Check sheet for the modelled part. Datum: model origin and axes. Units: mm. A direction names the side the tool comes from. Round coordinates to 2 decimals unless told otherwise and drop trailing zeros. Loops run counter-clockwise (first coordinate to the right, second up) from the corner with the lowest first, then second, coordinate; pieces in that order, holes last. Notation, with made-up numbers: (62.25, 62.25) - (79.25, 62.25) arc R28 ccw to (79.25, 91.25) - close; hole circle Ø3 at (71, 63.5). An arc over 180 degrees is marked (long way). Return JSON: item names as keys, results as strings.
from build123d import *

# Parameters (mm, degrees)
F0_W     = 45.085
F0_H     = 62.992
F1_DEPTH = 25.654
F2_R     = 2.286
F3_DEPTH = 35.306
F5_DEPTH = 21.209
F6_W     = 10.668
F6_H     = 7.9248
F7_DEPTH = 11.43
F8_W     = 10.668
F8_H     = 7.9248
F9_DEPTH = 11.43


with BuildPart() as f1:
    # F0 (on Front) → F1 (new body)
    with BuildSketch(Plane.XZ):
        Rectangle(F0_W, F0_H)
    extrude(amount=F1_DEPTH)

    # F2 (on face) → F3 (cut)
    with BuildSketch(Plane.XZ.offset(25.654)):
        with Locations((0, 23.876)):
            Circle(F2_R)
        with BuildLine():
            Line((-2.2225, -22.7965), (-2.2225, -25.4635))
            ThreePointArc((-2.2225, -25.4635), (0, -27.686), (2.2225, -25.4635))
            Line((2.2225, -25.4635), (2.2225, -22.7965))
            ThreePointArc((2.2225, -22.7965), (0, -20.574), (-2.2225, -22.7965))
        make_face()
    extrude(amount=-F3_DEPTH, mode=Mode.SUBTRACT)

    # F4 (on face) → F5 (cut)
    with BuildSketch(Plane.XZ.offset(25.654)):
        with BuildLine():
            Line((-5.08, 34.951579), (-5.08, 23.876))
            ThreePointArc((-5.08, 23.876), (0, 18.796), (5.08, 23.876))
            Line((5.08, 23.876), (5.08, 34.951579))
            Line((5.08, 34.951579), (-5.08, 34.951579))
        make_face()
        with BuildLine():
            Line((5.08, -34.4517), (5.08, -24.13))
            ThreePointArc((5.08, -24.13), (0, -19.05), (-5.08, -24.13))
            Line((-5.08, -24.13), (-5.08, -34.4517))
            Line((-5.08, -34.4517), (5.08, -34.4517))
        make_face()
    extrude(amount=-F5_DEPTH, mode=Mode.SUBTRACT)

    # F6 (on face) → F7 (cut)
    with BuildSketch(Plane(origin=(0, 0, -31.496), x_dir=(1, 0, 0), z_dir=(0, 0, -1))):
        with Locations((-13.716, 19.1516)):
            Rectangle(F6_W, F6_H)
        with Locations((13.716, 19.1516)):
            Rectangle(F6_W, F6_H)
    extrude(amount=-F7_DEPTH, mode=Mode.SUBTRACT)

    # F8 (on face) → F9 (cut)
    with BuildSketch(Plane.XY.offset(31.496)):
        with Locations((13.716, -19.1516)):
            Rectangle(F8_W, F8_H)
        with Locations((-13.716, -19.1516)):
            Rectangle(F8_W, F8_H)
    extrude(amount=-F9_DEPTH, mode=Mode.SUBTRACT)


solid = f1.part
Q1. Sectioned sample at C-C (x = 15). Enter the section's corners in (y, z).
Answer key:
{"outline": "(-25.65, -31.5) - (-23.11, -31.5) - (-23.11, -20.07) - (-15.19, -20.07) - (-15.19, -31.5) - (0, -31.5) - (0, 31.5) - (-15.19, 31.5) - (-15.19, 20.07) - (-23.11, 20.07) - (-23.11, 31.5) - (-25.65, 31.5) - close"}
Q2. Sectioned sample at D-D (y = -20.25). Enter the section's corners in (x, z).
Answer key:
{"outline": "(-22.54, -31.5) - (-19.05, -31.5) - (-19.05, -20.07) - (-8.38, -20.07) - (-8.38, -31.5) - (-5.08, -31.5) - (-5.08, -24.13) arc R5.08 cw to (5.08, -24.13) - (5.08, -31.5) - (8.38, -31.5) - (8.38, -20.07) - (19.05, -20.07) - (19.05, -31.5) - (22.54, -31.5) - (22.54, 31.5) - (19.05, 31.5) - (19.05, 20.07) - (8.38, 20.07) - (8.38, 31.5) - (5.08, 31.5) - (5.08, 23.88) arc R5.08 cw to (-5.08, 23.88) - (-5.08, 31.5) - (-8.38, 31.5) - (-8.38, 20.07) - (-19.05, 20.07) - (-19.05, 31.5) - (-22.54, 31.5) - close"}
Q3. Scan lines: probe 1 along Z at (x, y) = (0, -2.35); probe 2 along X at (y, z) = (-23, -25.5); probe 3 along X at (y, z) = (-5.75, 28.5). Record each from-to range of solid material in increasing order. Write a range as [from, to].
Answer key:
{"probe 1": "z = [-31.5, -27.69], [-20.57, 21.59], [26.16, 31.5]", "probe 2": "x = [-22.54, -19.05], [-8.38, -5.08], [5.08, 8.38], [19.05, 22.54]", "probe 3": "x = [-22.54, -5.08], [5.08, 22.54]"}
Q4. Sectioned sample at A-A (x = 0). Enter the section's corners in (y, z) (3 decimals).
Answer key:
{"outline": "(-25.654, -19.05) - (-4.445, -19.05) - (-4.445, -20.574) - (0, -20.574) - (0, 21.59) - (-4.445, 21.59) - (-4.445, 18.796) - (-25.654, 18.796) - close; (-4.445, -31.496) - (0, -31.496) - (0, -27.686) - (-4.445, -27.686) - close; (-4.445, 26.162) - (0, 26.162) - (0, 31.496) - (-4.445, 31.496) - close"}
Q5. Draft check along X on faces 1 (the face through (14, -23.114, 26)), 2 (the face through (0.049, -2.254, -20.575)). Enter one of: released by +X, released by -X, zero draft, split by the parting line, or undercut.
Answer key:
{"face 1": "undercut", "face 2": "undercut"}
Q6. Tool access check on faces 3 (the face through (0.11, -15.2, -19.05)), 4 (the face through (-0.112, -15.198, 18.797)), 5 (the face through (19.05, -19, 26)), 6 (the face through (14, -23.114, -26)). Record the directions out of +Z, -Z, +X, -X, +Y, -Y that give a thin tool (end or side, any length) a straight path to the whole face; none if there is none.
Answer key:
{"face 3": "-Z, -Y", "face 4": "+Z, -Y", "face 5": "+Z", "face 6": "-Z"}
Q7. Sectioned sample at B-B (y = -5.25). Enter the section's corners in (x, z), plus the area to 3 significant figures.
Answer key:
{"outline": "(-22.54, -31.5) - (-5.08, -31.5) - (-5.08, -24.13) arc R5.08 cw to (5.08, -24.13) - (5.08, -31.5) - (22.54, -31.5) - (22.54, 31.5) - (5.08, 31.5) - (5.08, 23.88) arc R5.08 cw to (-5.08, 23.88) - (-5.08, 31.5) - (-22.54, 31.5) - close", "area": "2,610 mm²"}
Q8. Depth check by flat-ended pin: P1, Ø11.5, axis at x = -14.5, z = 24.5, coming from the +Y side; P2, Ø5, axis at x = 2.5, z = 26, coming from the -Y side (3 decimals); P3, Ø2.5, axis at x = 13.5, y = -20, coming from the -Z side. Enter the tip coordinate at first touch or a pass-through.
Answer key:
{"P1": "stops at y = 0", "P2": "stops at y = -4.445", "P3": "stops at z = -20.07"}
